Work out the finished part from the listing and answer in its coordinate system (mm). Face numbers are marked on the shaded views. A direction names the side the tool comes from. Coordinates: 2 decimals unless noted, no trailing zeros. Loops run counter-clockwise (first coordinate to the right, second up) from the corner with the lowest first, then second, coordinate; pieces in that order, holes last. Notation, with made-up numbers: (9.25, 73.5) -> (67.25, 73.5) arc R19 ccw to (67.25, 83.5) -> close; hole circle Ø9 at (12, -26.75). An arc over 180 degrees is marked (long way). One line per question, with ' | ' between items.
```python
from build123d import *

# Parameters (mm, degrees)
BOSS_EXTRUDE1_DEPTH = 15.875
SKETCH2_W           = 3.87077
SKETCH2_H           = 7.9
BOSS_EXTRUDE2_DEPTH = 22.9
SKETCH3_W           = 3.175
SKETCH3_H           = 7.9
BOSS_EXTRUDE3_DEPTH = 12.7
SKETCH4_R           = 2.4003
CUT_EXTRUDE1_DEPTH  = 16.875


with BuildPart() as part:
    # Sketch1 → Boss-Extrude1 (new body)
    with BuildSketch(Plane.XY):
        Polygon((-96.811237268, -63.5), (-89.85, -63.5), (-89.85, -55.6), (-95.988636364, -55.6), (-96.811237268, -56.731076243), align=None)
    extrude(amount=BOSS_EXTRUDE1_DEPTH)

    # Sketch2 → Boss-Extrude2 (add)
    with BuildSketch(Plane(origin=(-89.85, 0, 0), x_dir=(0, 0, -1), z_dir=(1, 0, 0))):
        with Locations((-13.939615, -59.55)):
            Rectangle(SKETCH2_W, SKETCH2_H)
    extrude(amount=BOSS_EXTRUDE2_DEPTH)

    # Sketch3 → Boss-Extrude3 (add)
    with BuildSketch(Plane.XY.offset(15.875)):
        with Locations((-65.3625, -59.55)):
            Rectangle(SKETCH3_W, SKETCH3_H)
    extrude(amount=-BOSS_EXTRUDE3_DEPTH)

    # Sketch4 → Cut-Extrude1 (cut, through all)
    with BuildSketch(Plane.XY.offset(15.875)):
        with Locations((-93.032751555, -58.7375)):
            Circle(SKETCH4_R)
    extrude(amount=-CUT_EXTRUDE1_DEPTH, mode=Mode.SUBTRACT)


solid = part.part
```
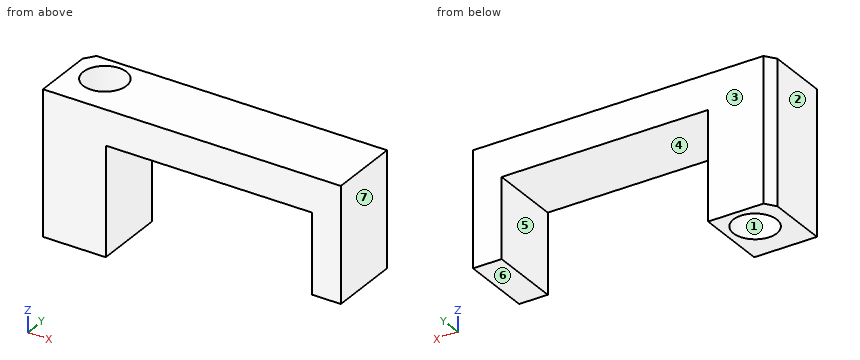
1) Find the intervals of material crossed by line 1 along X through (y, z) = (-57.25, 10.5) (3 decimals); line 2 along X through (y, z) = (-62, 9.75) (3 decimals); line 3 along X through (y, z) = (-60.5, 4.25) (3 decimals), in increasing order.
Check values:
line 1: x = -96.811 to -94.917, -91.149 to -89.85, -66.95 to -63.775 | line 2: x = -96.811 to -89.85, -66.95 to -63.775 | line 3: x = -96.811 to -94.662, -91.403 to -89.85, -66.95 to -63.775
2) Find section C-C (y = -60.5). Write down the section's boundary in (x, z) (3 decimals).
Check values:
outline: (-96.811, 0) -> (-94.662, 0) -> (-94.662, 15.875) -> (-96.811, 15.875) -> close; (-91.403, 0) -> (-89.85, 0) -> (-89.85, 12.004) -> (-66.95, 12.004) -> (-66.95, 3.175) -> (-63.775, 3.175) -> (-63.775, 15.875) -> (-91.403, 15.875) -> close
3) The mould has two halves that part along X. Classify the marked faces 1, 2, 3 and 4: released by +X, released by -X, zero draft, split by the parting line, or undercut.
Check values:
face 1: undercut | face 2: released by -X | face 3: zero draft | face 4: undercut
4) For the marked faces 5, 6 and 7, determine the directions among +Z, -Z, +X, -X, +Y, -Y from which every point of the face is accessible in a straight line to the end or side of a thin tool.
Check values:
face 5: -Z, +Y, -Y | face 6: -Z, +X, +Y, -Y | face 7: +Z, -Z, +X, +Y, -Y
5) Flat-ended cylindrical pins translate along their axes: pin 1 (2.5 mm diameter, centred on x = -74, y = -58.5, fed in from -Z); pin 2 (8 mm diameter, centred on x = -68.5, z = 9, fed in from -Y); pin 3 (1 mm diameter, centred on x = -66, y = -59, fed in from -Z) (3 decimals). Find the tip coordinate at first contact, or state that the pin passes through.
Check values:
pin 1: stops at z = 12 | pin 2: stops at y = -63.5 | pin 3: stops at z = 3.175
6) Find section B-B (x = -92). Write down the section's boundary in (y, z) (3 decimals).
Check values:
outline: (-63.5, 0) -> (-60.904, 0) -> (-60.904, 15.875) -> (-63.5, 15.875) -> close; (-56.571, 0) -> (-55.6, 0) -> (-55.6, 15.875) -> (-56.571, 15.875) -> close
7) Find section A-A (z = 3.5). State how many separate pieces and enclosed holes the cut face has, plus the area to 3 significant figures.
Check values:
separate pieces: 2 | enclosed holes: 1 | area: 61.5 mm^2
8) Find section D-D (y = -62). Write down the section's boundary in (x, z) (3 decimals).
Check values:
outline: (-96.811, 0) -> (-89.85, 0) -> (-89.85, 12.004) -> (-66.95, 12.004) -> (-66.95, 3.175) -> (-63.775, 3.175) -> (-63.775, 15.875) -> (-96.811, 15.875) -> close
